Job drawing, mm, ordinate dimensions from the low corner. One solid piece. Coordinates: 2 decimals unless noted, no trailing zeros. Write each loop counter-clockwise with the first axis right and the second up, starting at its lowest first coordinate (ties: lowest second). Pieces come first, ordered by that corner, then holes. Notation, with made-up numbers: M -20.5,81.25 L -2.5,81.25 A33 cw -2.5,112.25 Z; hole C -13.5,-36 d2. An arc over 180 degrees is marked long. Answer as CSV lines item,"result". Start each with the question number.
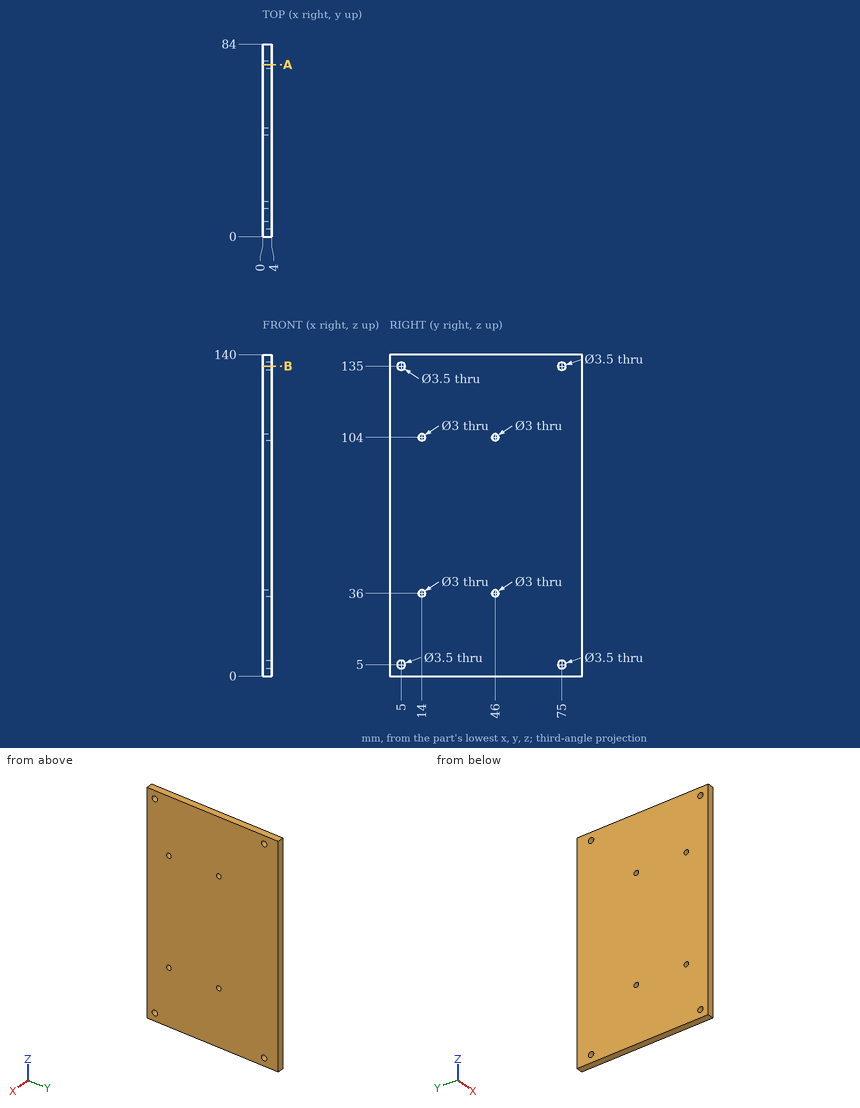
1) Band-saw the part on A-A, the plane y = 75. List the corners of the cut face in (x, z), plus the area to 3 significant figures.
2) Probe L1, parallel to Z at x = 1.65, y = 75; L2, parallel to Y at x = 1.7, z = 36; L3, parallel to Y at x = 0.95, z = 135. List the from-to ranges inside material, lowest first. Write a range as [from, to].
3) Band-saw the part on B-B, the plane z = 135. List the corners of the cut face in (x, y).
4) Pin check, flat tips, straight feed: P1, Ø2, axis at y = 5, z = 5, coming from the +X side; P2, Ø4.5, axis at y = 5, z = 135, coming from the +X side. Stop position of each tip, or through.
Result sheet:
1,outline,"M 0,0 L 4,0 L 4,3.25 L 0,3.25 Z; M 0,6.75 L 4,6.75 L 4,133.25 L 0,133.25 Z; M 0,136.75 L 4,136.75 L 4,140 L 0,140 Z"
1,area,"532 mm²"
2,L1,"z = [0, 3.25], [6.75, 133.25], [136.75, 140]"
2,L2,"y = [0, 12.5], [15.5, 44.5], [47.5, 84]"
2,L3,"y = [0, 3.25], [6.75, 73.25], [76.75, 84]"
3,outline,"M 0,0 L 4,0 L 4,3.25 L 0,3.25 Z; M 0,6.75 L 4,6.75 L 4,73.25 L 0,73.25 Z; M 0,76.75 L 4,76.75 L 4,84 L 0,84 Z"
4,P1,"passes through"
4,P2,"stops at x = 4"
